For this review, take the finished solid that the model builds, in its own axes (mm). Round coordinates to 2 decimals unless told otherwise and drop trailing zeros. Order: outer loops, then holes, each group sorted by start corner. A loop starts at its lowest first (then second) coordinate and runs counter-clockwise, first axis right, second up. Notation, with made-up numbers: M 84,-22 L 141,-22 A9 cw 141,-11 Z; hole C 32,19 d10. An arc over 180 degrees is marked long. Answer as a JSON object with one key per item and string values.
Autodesk Inventor part; units mm, degrees
ref_plane "YZ Plane" through (0, 0, 0) normal (1, 0, 0) x (0, 1, 0)
ref_plane "XZ Plane" through (0, 0, 0) normal (0, 1, 0) x (-1, 0, 0)
ref_plane "XY Plane" through (0, 0, 0) normal (0, 0, 1) x (1, 0, 0)
sketch "Sketch1" plane through (0, 0, 0) normal (0, 0, 1) x (1, 0, 0)
  line L0 (0, 0) -> (0, 38.1)
  line L1 (0, 38.1) -> (128.1684, 38.1)
  line L2 (128.1684, 38.1) -> (128.1684, 0)
  line L3 (128.1684, 0) -> (0, 0)
  dimension "d0" = 38.1
  dimension "d1" = 128.1684
extrude "Extrusion1" add sketch "Sketch1" along normal blind 3.175
sketch "Sketch2" plane through (0, 0, 3.175) normal (0, 0, 1) x (1, 0, 0)
  line L0 (128.1684, 38.1) -> (0, 38.1)
  line L1 (0, 38.1) -> (12.7, 38.1)
  line L2 (12.7, 38.1) -> (12.7, 31.75)
  line L3 (12.7, 31.75) -> (12.7, 6.35)
  circle A0 centre (12.7, 31.75) radius 3.3782
  circle A1 centre (12.7, 6.35) radius 3.3782
  line L4 (128.1684, 38.1) -> (115.4684, 38.1)
  line L5 (115.4684, 38.1) -> (115.4684, 31.75)
  circle A2 centre (115.4684, 31.75) radius 3.3782
  circle A3 centre (115.4684, 6.35) radius 3.3782
  line L6 (115.4684, 6.35) -> (115.4684, 31.75)
  dimension "d4" = 12.7
  dimension "d5" = 6.35
  dimension "d6" = 25.4
  dimension "d7" = 6.7564
  dimension "d8" = 6.7564
  dimension "d9" = 12.7
  dimension "d10" = 6.35
  dimension "d11" = 6.7564
  dimension "d12" = 6.7564
  dimension "d13" = 25.4
extrude "Extrusion2" cut sketch "Sketch2" against normal blind 3.175
fillet "Fillet1" radius 3.175 4 edges at (128.1684, 38.1, 1.5875) (128.1684, 0, 1.5875) (0, 38.1, 1.5875) (0, 0, 1.5875)
sketch "Sketch3" plane through (0, 0, 3.175) normal (0, 0, 1) x (1, 0, 0)
  arc A0 (0, 3.175) -> (3.175, 0) centre (3.175, 3.175) ccw
  line L0 (3.175, 0) -> (124.9934, 0)
  line L1 (124.9934, 38.1) -> (3.175, 38.1)
  arc A1 (3.175, 38.1) -> (0, 34.925) centre (3.175, 34.925) ccw
  line L2 (0, 34.925) -> (0, 3.175)
  circle A2 centre (12.7, 31.75) radius 3.3782
  circle A3 centre (12.7, 6.35) radius 3.3782
  line L3 (128.1684, 38.1) -> (102.7684, 38.1)
  line L4 (102.7684, 38.1) -> (102.7684, 0)
  point P0 (0, 0)
  dimension "d17" = 25.4
extrude "Extrusion3" cut sketch "Sketch3" against normal blind 25.4
fillet "Fillet2" radius 3.175 2 edges at (102.7684, 38.1, 1.5875) (102.7684, 0, 1.5875)
properties part number "spacer plate" material "Aluminum 6061"
1) Add section C-C on z = 1.85. State the section outline as (x, y) points (3 decimals), and give its area (3 significant figures).
Geometry check:
{"outline": "M 102.768,3.175 A3.175 ccw 105.943,0 L 124.993,0 A3.175 ccw 128.168,3.175 L 128.168,34.925 A3.175 ccw 124.993,38.1 L 105.943,38.1 A3.175 ccw 102.768,34.925 Z; hole C 115.468,6.35 d6.756; hole C 115.468,31.75 d6.756", "area": "887 mm²"}
2) Add section A-A on y = 31.75. State the section outline as (x, z) points (3 decimals).
Geometry check:
{"outline": "M 102.768,0 L 112.09,0 L 112.09,3.175 L 102.768,3.175 Z; M 118.847,0 L 128.168,0 L 128.168,3.175 L 118.847,3.175 Z"}
3) Add section B-B on x = 115.25. State the section outline as (y, z) points (3 decimals).
Geometry check:
{"outline": "M 0,0 L 2.979,0 L 2.979,3.175 L 0,3.175 Z; M 9.721,0 L 28.379,0 L 28.379,3.175 L 9.721,3.175 Z; M 35.121,0 L 38.1,0 L 38.1,3.175 L 35.121,3.175 Z"}
4) Mouldability with a two-part tool opening along X and no side actions: class faces 1 (the flat face through (115, 38.1, 2)), 2 (the cylindrical face through (112.093, 6.499, 1.61)), 3 (the cylindrical face through (103.674, 37.145, 1.565)) as +X half, -X half, draft (parallel to the pull), parting line (faces both ways), or undercut.
Geometry check:
{"face 1": "draft", "face 2": "undercut", "face 3": "-X half"}
5) Insertion check: P1, Ø9, axis at x = 115.47, y = 6.35, coming from the +Z side (3 decimals). The pin has a flat end and moves straight along its axis. Give the tip position at first contact, or say it passes through.
Geometry check:
{"P1": "stops at z = 3.175"}
6) For L1, parallel to X at y = 6.35, z = 1.6; L2, parallel to Y at x = 116.25, z = 1; L3, parallel to Y at x = 113.5, z = 0.4, list the stretches that pass through material, from the lowest coordinate up.
Geometry check:
{"L1": "x = 102.77 to 112.09, 118.85 to 128.17", "L2": "y = 0 to 3.06, 9.64 to 28.46, 35.04 to 38.1", "L3": "y = 0 to 3.6, 9.1 to 29, 34.5 to 38.1"}
